The model under review builds one solid part; all positions refer to its coordinate system, in mm. Round coordinates to 2 decimals unless told otherwise and drop trailing zeros. Order: outer loops, then holes, each group sorted by start corner. A loop starts at its lowest first (then second) coordinate and runs counter-clockwise, first axis right, second up. Notation, with made-up numbers: M 11.5,-37 L 56.5,-37 A21 cw 56.5,-8 Z; hole C -5,40 d1. An arc over 180 degrees is marked long. Answer as a JSON object with one key per item and string values. Group by question number.
1) Consider section A-A, the plane y = 10.5. Write out the cut boundary in (x, z), then the cut area to 3 significant figures.
2) Consider section D-D, the plane z = 1. Count the separate pieces of the cut face and the enclosed holes in it, then the cut area to 3 significant figures.
3) Consider section B-B, the plane x = 10. Write out the cut boundary in (y, z).
4) Consider section C-C, the plane x = 37.6. Write out the cut boundary in (y, z), then the cut area to 3 significant figures.
5) To check wall thickness, follow line 1 (Y direction, x = 37.6, z = 1); line 2 (Y direction, x = 58, z = 1.95); line 3 (X direction, y = 0, z = 0.6). State the ranges of each line that lie inside material, in increasing order.
6) Insertion check: pin 1 Ø1.5 at (y, z) = (-3.5, 2) entering from +X; pin 2 Ø1.8 at (x, y) = (37.6, 22.9) entering from +Z. Each pin has a flat end and moves straight along its axis. Give the tip position at first contact, or say it passes through.
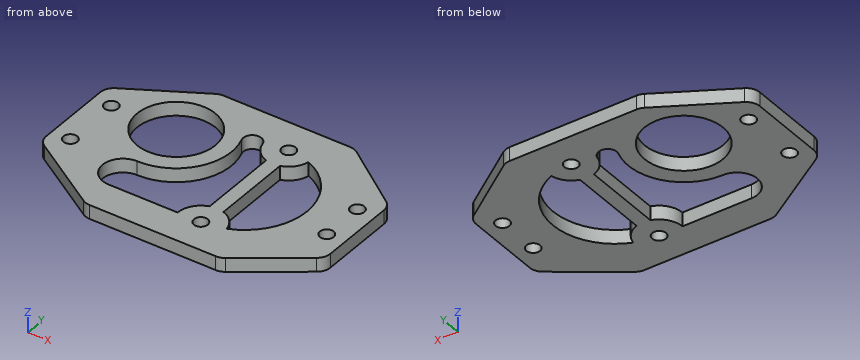
```python
from build123d import *

# Parameters (mm, degrees)
SKETCH1_R           = 1.5
SKETCH1_R_2         = 8.5
BOSS_EXTRUDE1_DEPTH = 3


with BuildPart() as part:
    # Sketch1 → Boss-Extrude1 (new body)
    with BuildSketch(Plane.XY):
        with BuildLine():
            Line((0, 1.64796966), (0, 18.25796966))
            ThreePointArc((0, 18.25796966), (0.407702513, 19.767934474), (1.519995827, 20.867488322))
            Line((1.519995827, 20.867488322), (16.942251121, 29.614312984))
            ThreePointArc((16.942251121, 29.614312984), (17.656930521, 29.905531813), (18.422255294, 30.004794322))
            Line((18.422255294, 30.004794322), (45.922255294, 30.004794322))
            ThreePointArc((45.922255294, 30.004794322), (46.845265991, 29.859273478), (47.678731824, 29.43682849))
            Line((47.678731824, 29.43682849), (60.756476531, 19.991750808))
            ThreePointArc((60.756476531, 19.991750808), (61.671088691, 18.925471084), (62, 17.559716639))
            Line((62, 17.559716639), (62, 1.129716639))
            ThreePointArc((62, 1.129716639), (61.66533053, -0.247241299), (60.735991224, -1.316982049))
            Line((60.735991224, -1.316982049), (47.579391193, -10.651904367))
            ThreePointArc((47.579391193, -10.651904367), (46.754416966, -11.063535266), (45.84339997, -11.205205678))
            Line((45.84339997, -11.205205678), (18.50339997, -11.205205678))
            ThreePointArc((18.50339997, -11.205205678), (17.66547208, -11.085809235), (16.894241264, -10.73712358))
            Line((16.894241264, -10.73712358), (1.390841294, -0.883948242))
            ThreePointArc((1.390841294, -0.883948242), (0.370601198, 0.203579844), (0, 1.64796966))
        make_face()
        with Locations((4, 16.007488322)):
            Circle(SKETCH1_R, mode=Mode.SUBTRACT)
        with Locations((4, 3.4375)):
            Circle(SKETCH1_R, mode=Mode.SUBTRACT)
        with Locations((58, 15.091750808)):
            Circle(SKETCH1_R, mode=Mode.SUBTRACT)
        with Locations((58, 5.678289269)):
            Circle(SKETCH1_R, mode=Mode.SUBTRACT)
        with Locations((37.6, 22.899794322)):
            Circle(SKETCH1_R, mode=Mode.SUBTRACT)
        with Locations((37.6, -4.100205678)):
            Circle(SKETCH1_R, mode=Mode.SUBTRACT)
        with Locations((17.6, 16.679794322)):
            Circle(SKETCH1_R_2, mode=Mode.SUBTRACT)
        with BuildLine():
            Line((39.1, 0.713961497), (39.1, 18.085627146))
            ThreePointArc((39.1, 18.085627146), (41.365876, 19.546529711), (42.555224583, 21.966009055))
            ThreePointArc((42.555224583, 21.966009055), (51.107923726, 9.399794322), (42.555224583, -3.166420412))
            ThreePointArc((42.555224583, -3.166420412), (41.365876, -0.746941068), (39.1, 0.713961497))
        make_face(mode=Mode.SUBTRACT)
        with BuildLine():
            Line((36.1, 18.085627146), (36.1, 0.713961497))
            ThreePointArc((36.1, 0.713961497), (33.538604534, -1.111682219), (32.55755956, -4.100205678))
            Line((32.55755956, -4.100205678), (17.6, -4.100205678))
            ThreePointArc((17.6, -4.100205678), (13.21, 0.289794322), (17.6, 4.679794322))
            ThreePointArc((17.6, 4.679794322), (27.411976087, 9.771456948), (28.897406852, 20.725606777))
            ThreePointArc((28.897406852, 20.725606777), (30.206772534, 23.282822768), (32.675850225, 21.813997568))
            ThreePointArc((32.675850225, 21.813997568), (33.886159456, 19.488988843), (36.1, 18.085627146))
        make_face(mode=Mode.SUBTRACT)
    extrude(amount=BOSS_EXTRUDE1_DEPTH)


solid = part.part
```
Results list:
{
 "1": {"outline": "M 0,0 L 11.76,0 L 11.76,3 L 0,3 Z; M 23.44,0 L 27.89,0 L 27.89,3 L 23.44,3 Z; M 36.1,0 L 39.1,0 L 39.1,3 L 36.1,3 Z; M 51.06,0 L 62,0 L 62,3 L 51.06,3 Z", "area": "90.5 mm^2"},
 "2": {"separate pieces": "1", "enclosed holes": "9", "area": "1,390 mm^2"},
 "3": {"outline": "M -6.36,0 L 12.87,0 L 12.87,3 L -6.36,3 Z; M 20.49,0 L 25.68,0 L 25.68,3 L 20.49,3 Z"},
 "4": {"outline": "M -11.21,0 L -5.6,0 L -5.6,3 L -11.21,3 Z; M -2.6,0 L 21.4,0 L 21.4,3 L -2.6,3 Z; M 24.4,0 L 30,0 L 30,3 L 24.4,3 Z", "area": "106 mm^2"},
 "5": {"line 1": "-11.21 to -5.6, -2.6 to 21.4, 24.4 to 30", "line 2": "-3.26 to 4.18, 7.18 to 13.59, 16.59 to 21.98", "line 3": "0.49 to 13.22, 34.66 to 40.54, 47.3 to 61.78"},
 "6": {"pin 1": "x = 58.72", "pin 2": "through"}
}
